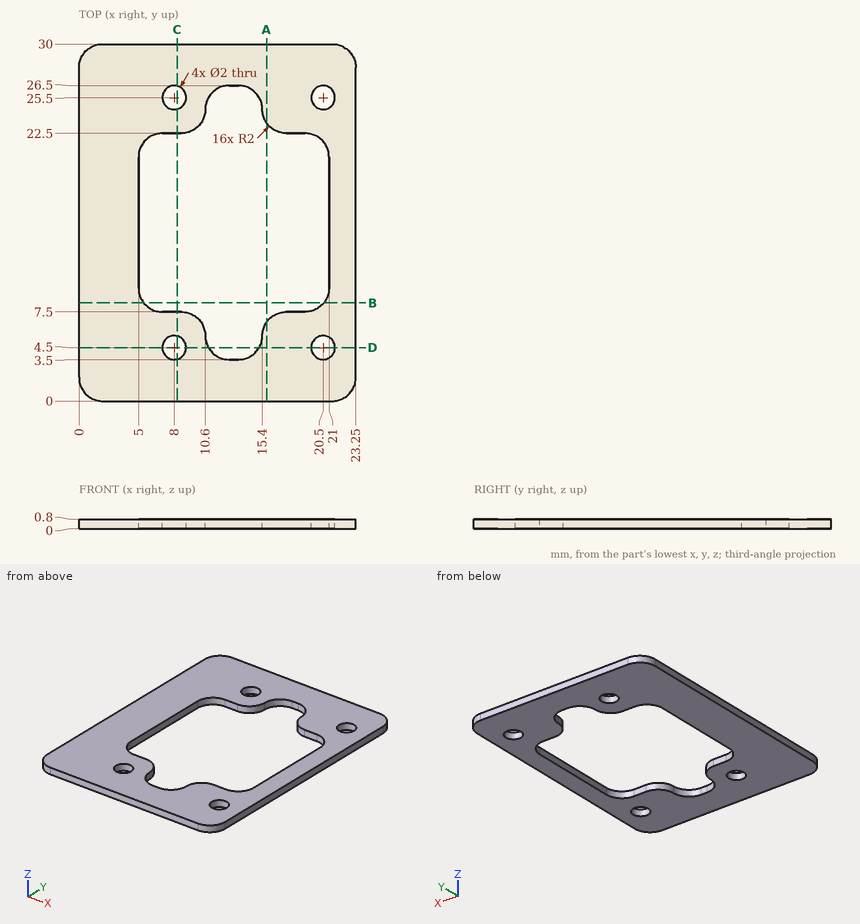
Geometry check sheet. Reference: drawing and pictorial views, mm from the part's lowest x, y, z. Round coordinates to 2 decimals unless told otherwise and drop trailing zeros. Loops run counter-clockwise (first coordinate to the right, second up) from the corner with the lowest first, then second, coordinate; pieces in that order, holes last. Notation, with made-up numbers: (37.25, 83) -> (68.25, 83) arc R12 ccw to (68.25, 103) -> close; hole circle Ø4 at (61.25, 33). An arc over 180 degrees is marked (long way). Answer as a JSON object with one key per item and string values.
Q1. Go/stop test with a flat-tipped pin: P1, Ø1, axis at x = 8, y = 25.5, coming from the +Z side. Record where the tip stops, or that it passes through.
Data:
{"P1": "passes through"}
Q2. Section check B-B (y = 8.25). Record the boundary of the cut face in (x, z).
Data:
{"outline": "(0, 0) -> (5.44, 0) -> (5.44, 0.8) -> (0, 0.8) -> close; (20.56, 0) -> (23.25, 0) -> (23.25, 0.8) -> (20.56, 0.8) -> close"}
Q3. Section check D-D (y = 4.5). Record the boundary of the cut face in (x, z), then the cut area to 3 significant figures.
Data:
{"outline": "(0, 0) -> (7, 0) -> (7, 0.8) -> (0, 0.8) -> close; (9, 0) -> (10.87, 0) -> (10.87, 0.8) -> (9, 0.8) -> close; (15.13, 0) -> (19.5, 0) -> (19.5, 0.8) -> (15.13, 0.8) -> close; (21.5, 0) -> (23.25, 0) -> (23.25, 0.8) -> (21.5, 0.8) -> close", "area": "12.0 mm2"}
Q4. Section check C-C (x = 8.25). Record the boundary of the cut face in (y, z).
Data:
{"outline": "(0, 0) -> (3.53, 0) -> (3.53, 0.8) -> (0, 0.8) -> close; (5.47, 0) -> (7.5, 0) -> (7.5, 0.8) -> (5.47, 0.8) -> close; (22.5, 0) -> (24.53, 0) -> (24.53, 0.8) -> (22.5, 0.8) -> close; (26.47, 0) -> (30, 0) -> (30, 0.8) -> (26.47, 0.8) -> close"}
Q5. Section check A-A (x = 15.75). Record the boundary of the cut face in (y, z), then the cut area to 3 significant figures.
Data:
{"outline": "(0, 0) -> (6.63, 0) -> (6.63, 0.8) -> (0, 0.8) -> close; (23.37, 0) -> (30, 0) -> (30, 0.8) -> (23.37, 0.8) -> close", "area": "10.6 mm2"}
Q6. Scan lines: line 1 (Y direction, x = 8, z = 0.35); line 2 (Y direction, x = 20.5, z = 0.6); line 3 (X direction, y = 3.75, z = 0.15). Record each from-to range of solid material in increasing order. Write a range as from..to.
Data:
{"line 1": "y = 0..3.5, 5.5..7.5, 22.5..24.5, 26.5..30", "line 2": "y = 0..3.5, 5.5..8.18, 21.82..24.5, 26.5..30", "line 3": "x = 0..7.34, 8.66..11.63, 14.37..19.84, 21.16..23.25"}
